Read the model definition and answer for the solid it produces. Units are mm, in the model's axes. Face numbers are marked on the shaded views. A direction names the side the tool comes from. Give positions to 0.01 mm unless a question says otherwise; leave off trailing zeros. Loops run counter-clockwise (first coordinate to the right, second up) from the corner with the lowest first, then second, coordinate; pieces in that order, holes last.
(1) Find section D-D, the plane y = 8. Write down the section's boundary in (x, z) (3 decimals), then the cut area to 3 significant figures.
(2) Straight lines are drawn through the part: probe 1 along Y at (x, z) = (6.35, 9.5); probe 2 along Y at (x, z) = (16, 23.5); probe 3 along Y at (x, z) = (5.5, 8). For each, find the intervals that lie inside material, in ascending order.
(3) Which of the six approach directions +Z, -Z, +X, -X, +Y, -Y give full straight-line access (tool end or side, diameter ignored) to the marked faces 5 and 6?
(4) Find section B-B, the plane z = 35. Write down the section's boundary in (x, y), then the cut area to 3 significant figures.
(5) Each of these flat-tipped pins is pushed along its axis until it touches: P1, Ø3, axis at x = 17, y = 16, coming from the +Z side; P2, Ø3, axis at x = 6.35, y = 4.78, coming from the -Z side; P3, Ø1, axis at y = 22.5, z = 19, coming from the -X side. Where does it stop, or does it pass through?
(6) Find section A-A, the plane z = 25.4. Write down the section's boundary in (x, y), then the cut area to 3 significant figures.
(7) Find section C-C, the plane x = 7.25. Write down the section's boundary in (y, z), then the cut area to 3 significant figures.
(8) Determine the mould class of the marked faces 1, 2, 3 and 4 for opening direction Y: pulls with the +Y half, pulls with the -Y half, needs draft (parallel to the pull), parting line crosses it, or undercut.
```python
from build123d import *

# Parameters (mm, degrees)
F1_DEPTH = 19.05
F2_R     = 3.175
F3_DEPTH = 76.2
F4_R     = 1.679652
F5_DEPTH = 12.7


with BuildPart() as f1:
    # F0 (on Right) → F1 (new body)
    with BuildSketch(Plane.YZ):
        Polygon((11.43, 38.1), (0, 38.1), (0, 0), (35.56, 0), (35.56, 38.1), (24.13, 38.1), (24.13, 6.35), (11.43, 6.35), align=None)
    extrude(amount=F1_DEPTH)

    # F2 (on face) → F3 (cut)
    with BuildSketch(Plane.XZ):
        with Locations((9.525, 25.4)):
            Circle(F2_R)
    extrude(amount=-F3_DEPTH, mode=Mode.SUBTRACT)

    # F4 (on face) → F5 (cut)
    with BuildSketch(Plane(origin=(0, 0, 0), x_dir=(1, 0, 0), z_dir=(0, 0, -1))):
        with Locations((6.35, -4.7752)):
            Circle(F4_R)
        with Locations((6.35, -30.7848)):
            Circle(F4_R)
    extrude(amount=-F5_DEPTH, mode=Mode.SUBTRACT)


solid = f1.part
```
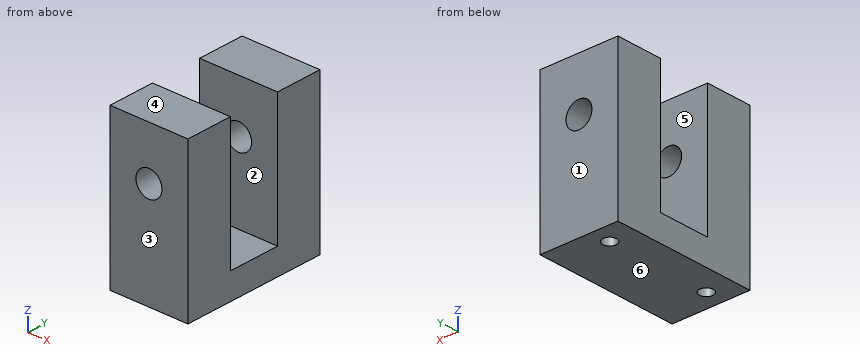
Entries:
1. outline: (0, 0) - (19.05, 0) - (19.05, 38.1) - (0, 38.1) - close; hole circle Ø6.35 at (9.525, 25.4)
1. area: 694 mm2
2. probe 1: y = 0 to 3.1, 6.45 to 11.43, 24.13 to 29.11, 32.46 to 35.56
2. probe 2: y = 0 to 11.43, 24.13 to 35.56
2. probe 3: y = 0 to 3.33, 6.22 to 11.43, 24.13 to 29.34, 32.23 to 35.56
3. face 5: +Z, +X, -X
3. face 6: -Z, +X, -X, +Y, -Y
4. outline: (0, 0) - (19.05, 0) - (19.05, 11.43) - (0, 11.43) - close; (0, 24.13) - (19.05, 24.13) - (19.05, 35.56) - (0, 35.56) - close
4. area: 435 mm2
5. P1: stops at z = 6.35
5. P2: stops at z = 12.7
5. P3: passes through
6. outline: (0, 0) - (6.35, 0) - (6.35, 11.43) - (0, 11.43) - close; (0, 24.13) - (6.35, 24.13) - (6.35, 35.56) - (0, 35.56) - close; (12.7, 0) - (19.05, 0) - (19.05, 11.43) - (12.7, 11.43) - close; (12.7, 24.13) - (19.05, 24.13) - (19.05, 35.56) - (12.7, 35.56) - close
6. area: 290 mm2
7. outline: (0, 0) - (3.36, 0) - (3.36, 12.7) - (6.19, 12.7) - (6.19, 0) - (29.37, 0) - (29.37, 12.7) - (32.2, 12.7) - (32.2, 0) - (35.56, 0) - (35.56, 23.19) - (24.13, 23.19) - (24.13, 6.35) - (11.43, 6.35) - (11.43, 23.19) - (0, 23.19) - close; (0, 27.61) - (11.43, 27.61) - (11.43, 38.1) - (0, 38.1) - close; (24.13, 27.61) - (35.56, 27.61) - (35.56, 38.1) - (24.13, 38.1) - close
7. area: 778 mm2
8. face 1: pulls with the +Y half
8. face 2: undercut
8. face 3: pulls with the -Y half
8. face 4: needs draft
